Build history of the part. All positions in model axes, mm. Face numbers are marked on the shaded views. A direction names the side the tool comes from. Coordinates: 2 decimals unless noted, no trailing zeros. Loops run counter-clockwise (first coordinate to the right, second up) from the corner with the lowest first, then second, coordinate; pieces in that order, holes last. Notation, with made-up numbers: M 3,88 L 37,88 A17 cw 37,95 Z; hole C -31.5,69.25 d7. An arc over 180 degrees is marked long. Write each question's results on one line, items separated by ' | '. Start each with the question number.
from build123d import *

# Parameters (mm, degrees)
BOSS_EXTRUDE1_DEPTH = 3
BOSS_EXTRUDE2_DEPTH = 6
SKETCH3_W           = 2
SKETCH3_H           = 1
CUT_EXTRUDE1_DEPTH  = 6


with BuildPart() as part:
    # Sketch1 → Boss-Extrude1 (new body)
    with BuildSketch(Plane.XY):
        Polygon((3, 0), (-3, 0), (-3, 2), (0, 5), (3, 2), align=None)
    extrude(amount=-BOSS_EXTRUDE1_DEPTH)

    # Sketch2 → Boss-Extrude2 (add)
    with BuildSketch(Plane(origin=(3, 0, 0), x_dir=(0, 0, -1), z_dir=(1, 0, 0))):
        Polygon((0, 3), (-3.04018422, 0), (0, 0), align=None)
    extrude(amount=-BOSS_EXTRUDE2_DEPTH)

    # Sketch3 → Cut-Extrude1 (cut)
    with BuildSketch(Plane.XY):
        Polygon((-2, 3), (-3, 2), (-3, 3), align=None)
        Polygon((2, 3), (3, 2), (3, 3), align=None)
        with Locations((0, 0.5)):
            Rectangle(SKETCH3_W, SKETCH3_H)
    extrude(amount=CUT_EXTRUDE1_DEPTH, mode=Mode.SUBTRACT)


solid = part.part
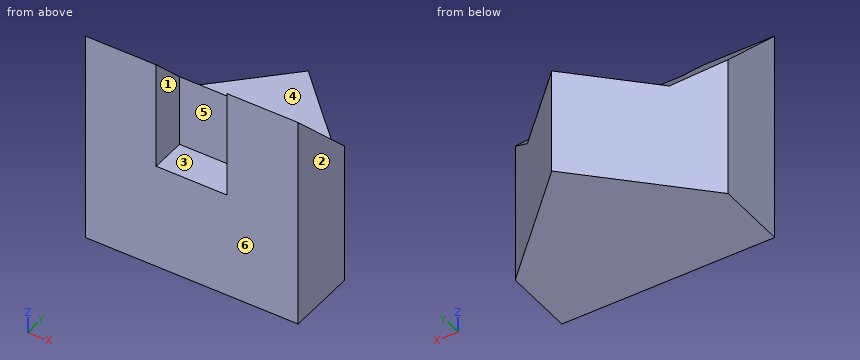
1. Band-saw the part on A-A, the plane x = 0.45. List the corners of the cut face in (y, z), plus the area to 3 significant figures.
2. Band-saw the part on B-B, the plane z = 2.5. List the corners of the cut face in (x, y), plus the area to 3 significant figures.
3. Band-saw the part on C-C, the plane y = 0.8. List the corners of the cut face in (x, z), plus the area to 3 significant figures.
4. Mould opens along X. For the marked faces 1, 2, 3 and 4 say: +X half, -X half, draft (parallel to the pull), parting line (faces both ways), or undercut.
5. Which spindle directions (+Z, -Z, +X, -X, +Y, -Y) get a long thin tool onto all of the face, cutting with end or side? Do the marked faces 5 and 6. Say none if no direction does.
6. Band-saw the part on D-D, the plane z = -0.5. List the corners of the cut face in (x, y).
7. Wall check: line 1 along Z through (x, y) = (0.05, 0.8); line 2 along Y through (x, z) = (1.25, -1); line 3 along Y through (x, z) = (-0.75, 0.75). Give the ranges that are in metal, low to high.
8. Pin check, flat tips, straight feed: pin 1 (1.5 mm diameter, centred on y = 3, z = -1, fed in from -X); pin 2 (1 mm diameter, centred on y = 4, z = 2, fed in from -X); pin 3 (1.5 mm diameter, centred on x = -2, z = -0.5, fed in from +Y); pin 4 (0.6 mm diameter, centred on x = 0, z = 1.5, fed in from -Y). Stop position of each tip, or through.
Checked values:
1) outline: M 0,-3 L 4.55,-3 L 4.55,0 L 3,0 L 1,2.03 L 1,0 L 0,0 Z | area: 15.7 mm²
2) outline: M -3,0 L -1,0 L -1,0.53 L -3,0.53 Z; M 1,0 L 3,0 L 3,0.53 L 1,0.53 Z | area: 2.13 mm²
3) outline: M -3,-3 L 3,-3 L 3,2.23 L 1,2.23 L 1,0 L -1,0 L -1,2.23 L -3,2.23 Z | area: 26.9 mm²
4) face 1: undercut | face 2: +X half | face 3: undercut | face 4: draft
5) face 5: +Z, -Y | face 6: +Z, -Z, +X, -X, -Y
6) outline: M -3,0 L 3,0 L 3,2 L 0,5 L -3,2 Z
7) line 1: -3 to 0 | line 2: 0 to 3.75 | line 3: 1 to 2.26
8) pin 1: x = -2.75 | pin 2: through | pin 3: y = 3.75 | pin 4: y = 1
